```python
from build123d import *

# Parameters (mm, degrees)
SKETCH_1_W          = 25
SKETCH_1_H          = 22
SKETCH_1_R          = 1.5
EXTRUDE_1_DEPTH     = 4
SKETCH_2_W          = 25
SKETCH_2_H          = 10
CUT_EXTRUDE_1_DEPTH = 0.8


with BuildPart() as part:
    # 草图1 → 凸台-拉伸1 (new body)
    with BuildSketch(Plane.XY):
        Rectangle(SKETCH_1_W, SKETCH_1_H)
        with Locations((-9.5, 7)):
            Circle(SKETCH_1_R, mode=Mode.SUBTRACT)
        with Locations((9.5, 7)):
            Circle(SKETCH_1_R, mode=Mode.SUBTRACT)
        with Locations(Location((9.5, -7, 0), (0, 0, 180))):
            Circle(SKETCH_1_R, mode=Mode.SUBTRACT)
        with Locations(Location((-9.5, -7, 0), (0, 0, 180))):
            Circle(SKETCH_1_R, mode=Mode.SUBTRACT)
    extrude(amount=EXTRUDE_1_DEPTH)

    # 草图2 → 切除-拉伸1 (cut)
    with BuildSketch(Plane.XY.offset(4)):
        Rectangle(SKETCH_2_W, SKETCH_2_H)
    extrude(amount=-CUT_EXTRUDE_1_DEPTH, mode=Mode.SUBTRACT)


solid = part.part
```
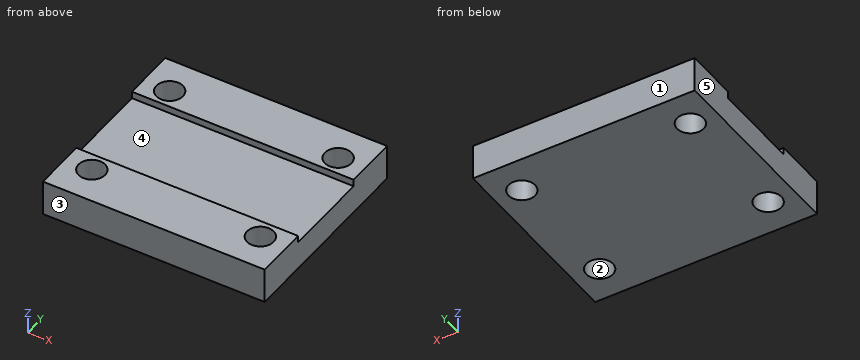
The model under review builds one solid part; all positions refer to its coordinate system, in mm. Face numbers are marked on the shaded views. A direction names the side the tool comes from. Round coordinates to 2 decimals unless told otherwise and drop trailing zeros. Order: outer loops, then holes, each group sorted by start corner. A loop starts at its lowest first (then second) coordinate and runs counter-clockwise, first axis right, second up. Notation, with made-up numbers: (-15, 61.25) -> (8, 61.25) arc R23 ccw to (8, 93.25) -> close; hole circle Ø1 at (12.5, -32). An arc over 180 degrees is marked (long way). One line per item, written item: value. Start each with the question number.
Q1. Take a section at C-C (x = 9.5). Write out the cut boundary in (y, z), and give its area (3 significant figures).
Q2. Mouldability with a two-part tool opening along Y and no side actions: class the marked faces 1, 2 and 3 as released by +Y, released by -Y, zero draft, split by the parting line, or undercut.
Q3. Machinability: for the marked faces 4 and 5, which of the approach directions +Z, -Z, +X, -X, +Y, -Y give a long, thin tool a straight path to every point of the face, cutting with its end or side? Answer none if there is none.
Q4. Take a section at B-B (y = 7). Write out the cut boundary in (x, z), and give its area (3 significant figures).
Q5. Wall thickness on line 1 (X direction, y = -7, z = 2.1); line 2 (Y direction, x = 1.75, z = 3.7); line 3 (Y direction, x = 9.5, z = 0.8): over which ranges is each line inside the solid? List them lowest first.
Q6. Take a section at D-D (z = 1.25). Write out the cut boundary in (x, y).
Q7. Take a section at A-A (z = 3.7). Write out the cut boundary in (x, y), and give its area (3 significant figures).
Q8. Clearance check with flat-ended pins moving along their axes: pin 1 Ø3 at (x, y) = (-4, 1.5) entering from +Z; pin 2 Ø2.5 at (x, y) = (9.5, -7) entering from -Z. State where each tip first meets the part, or that it passes through.
Reported:
1. outline: (-11, 0) -> (-8.5, 0) -> (-8.5, 4) -> (-11, 4) -> close; (-5.5, 0) -> (5.5, 0) -> (5.5, 4) -> (5, 4) -> (5, 3.2) -> (-5, 3.2) -> (-5, 4) -> (-5.5, 4) -> close; (8.5, 0) -> (11, 0) -> (11, 4) -> (8.5, 4) -> close
1. area: 56.0 mm2
2. face 1: released by +Y
2. face 2: undercut
2. face 3: released by -Y
3. face 4: +Z, +X, -X
3. face 5: +Z, -Z, -X, +Y, -Y
4. outline: (-12.5, 0) -> (-11, 0) -> (-11, 4) -> (-12.5, 4) -> close; (-8, 0) -> (8, 0) -> (8, 4) -> (-8, 4) -> close; (11, 0) -> (12.5, 0) -> (12.5, 4) -> (11, 4) -> close
4. area: 76.0 mm2
5. line 1: x = -12.5 to -11, -8 to 8, 11 to 12.5
5. line 2: y = -11 to -5, 5 to 11
5. line 3: y = -11 to -8.5, -5.5 to 5.5, 8.5 to 11
6. outline: (-12.5, -11) -> (12.5, -11) -> (12.5, 11) -> (-12.5, 11) -> close; hole circle Ø3 at (-9.5, -7); hole circle Ø3 at (-9.5, 7); hole circle Ø3 at (9.5, -7); hole circle Ø3 at (9.5, 7)
7. outline: (-12.5, -11) -> (12.5, -11) -> (12.5, -5) -> (-12.5, -5) -> close; (-12.5, 5) -> (12.5, 5) -> (12.5, 11) -> (-12.5, 11) -> close; hole circle Ø3 at (-9.5, -7); hole circle Ø3 at (-9.5, 7); hole circle Ø3 at (9.5, -7); hole circle Ø3 at (9.5, 7)
7. area: 272 mm2
8. pin 1: stops at z = 3.2
8. pin 2: passes through
